Drawing for the job (mm, zero at the part's lowest x, y, z). Round coordinates to 2 decimals unless told otherwise and drop trailing zeros. Loops run counter-clockwise (first coordinate to the right, second up) from the corner with the lowest first, then second, coordinate; pieces in that order, holes last. Notation, with made-up numbers: (58, 13.5) -> (110, 13.5) arc R30 ccw to (110, 35.5) -> close; hole circle Ø8 at (-34, 14). An arc over 180 degrees is marked (long way). Put each result on its own line as item: value. Start each with the question number.
Item 1: Drill centre lines: probe 1 along Y at (x, z) = (198.12, 2) (1 decimal); probe 2 along Y at (x, z) = (11.5, 3.25); probe 3 along X at (y, z) = (175.5, 4.25). Where is each one in solid material? Low to high. Write a range as [from, to].
Item 2: Cut at D-D, the plane y = 31.5. List the corners of the cut face in (x, z).
Item 3: Flat gauge pin, fed straight in: pin 1 Ø1.9 at (x, z) = (15, 2.5) entering from -Y. Where does the tip first touch, or does it go through?
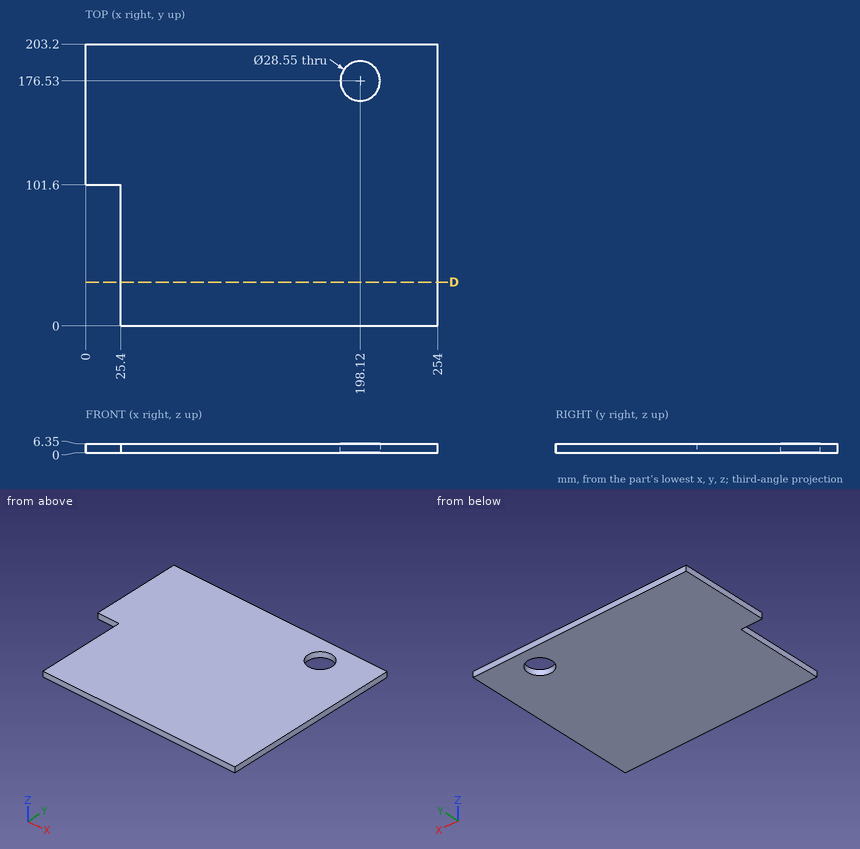
Reply:
1. probe 1: y = [0, 162.3], [190.8, 203.2]
1. probe 2: y = [101.6, 203.2]
1. probe 3: x = [0, 183.88], [212.36, 254]
2. outline: (25.4, 0) -> (254, 0) -> (254, 6.35) -> (25.4, 6.35) -> close
3. pin 1: stops at y = 101.6
